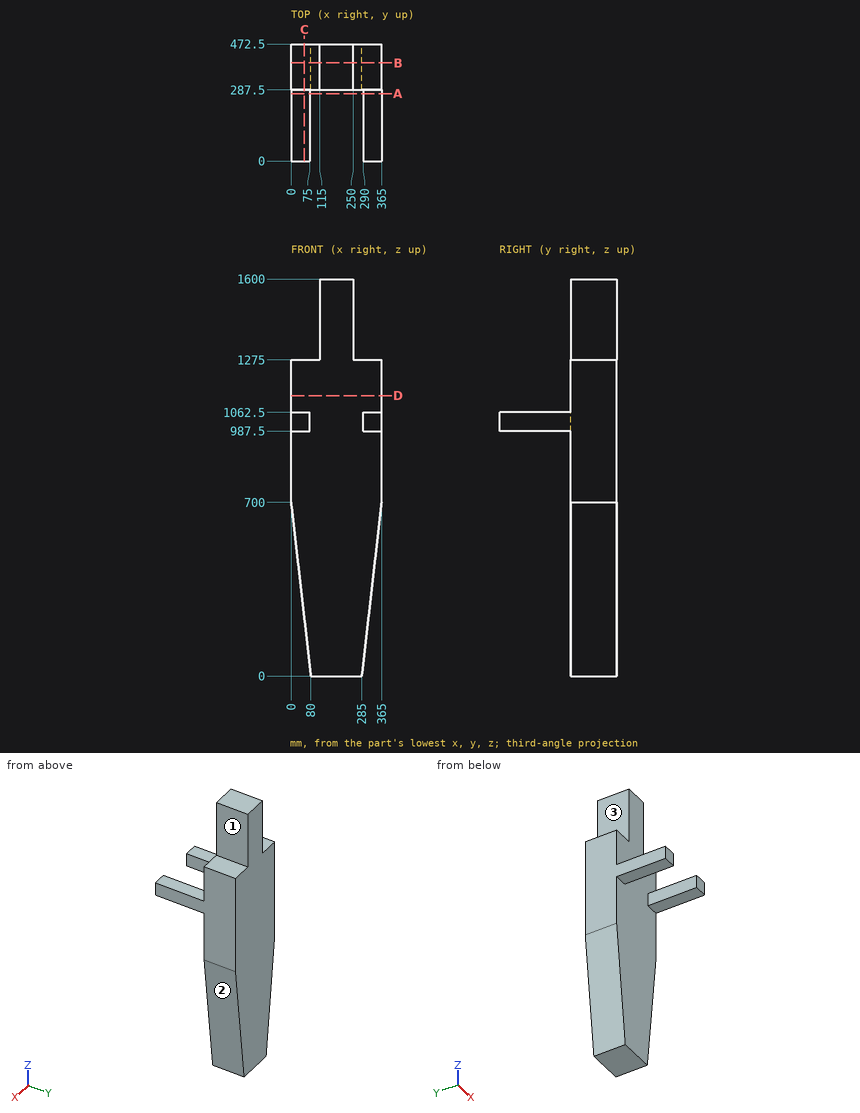
Input: dimensioned drawing with shaded views. Units: mm. Origin: part minimum x, y, z. A direction names the side the tool comes from. Round coordinates to 2 decimals unless told otherwise and drop trailing zeros. Write each loop counter-clockwise with the first axis right and the second up, starting at its lowest first coordinate (ties: lowest second). Pieces come first, ordered by that corner, then holes. Notation, with made-up numbers: (-30, -12.5) -> (-13, -12.5) arc R20 cw to (-13, 5.5) -> close; hole circle Ø11 at (-8.5, 15.25). An arc over 180 degrees is marked (long way). Use CSV: the item, a comma, the result in double quotes. Start each with the question number.
Q1. Section D-D (z = 1131). Return loops of the section in (x, y).
Q2. First-contact query: pin 1 Ø6 at (x, z) = (47.5, 1102.5) entering from -Y; pin 2 Ø5 at (x, y) = (59, 114.5) entering from -Z. Flat tips, straight axial feed; report the tip coordinate or a pass-through.
Q3. Line query: L1, parallel to Y at x = 97.5, z = 94; L2, parallel to X at y = 325.5, z = 1511; L3, parallel to Z at x = 62, y = 150.5. Output: solid intervals per line, ascending.
Q4. Section A-A (y = 272). Return loops of the section in (x, z).
Q5. Reachability of the marked faces 1, 2 and 3 from +Z, -Z, +X, -X, +Y, -Y: full face, straight path, thin tool, end or side. Return the list, or none.
Q6. Section B-B (y = 396). Return loops of the section in (x, z).
Q7. Section C-C (x = 53). Return loops of the section in (y, z).
Result sheet:
1,outline,"(0, 287.5) -> (365, 287.5) -> (365, 472.5) -> (0, 472.5) -> close"
2,pin 1,"y = 287.5"
2,pin 2,"z = 987.5"
3,L1,"287.5 to 472.5"
3,L2,"115 to 250"
3,L3,"987.5 to 1062.5"
4,outline,"(0, 987.5) -> (75, 987.5) -> (75, 1062.5) -> (0, 1062.5) -> close; (290, 987.5) -> (365, 987.5) -> (365, 1062.5) -> (290, 1062.5) -> close"
5,face 1,"+Z, +X, +Y, -Y"
5,face 2,"-Z, +X, +Y, -Y"
5,face 3,"+Z, -X, +Y, -Y"
6,outline,"(0, 700) -> (80, 0) -> (285, 0) -> (365, 700) -> (365, 1275) -> (250, 1275) -> (250, 1600) -> (115, 1600) -> (115, 1275) -> (0, 1275) -> close"
7,outline,"(0, 987.5) -> (287.5, 987.5) -> (287.5, 236.25) -> (472.5, 236.25) -> (472.5, 1275) -> (287.5, 1275) -> (287.5, 1062.5) -> (0, 1062.5) -> close"
